Model file for the job. Use its own axes, mm. A direction names the side the tool comes from. Round coordinates to 2 decimals unless told otherwise and drop trailing zeros. Loops run counter-clockwise (first coordinate to the right, second up) from the corner with the lowest first, then second, coordinate; pieces in that order, holes last. Notation, with made-up numbers: M 69.5,34 L 105.5,34 A16 cw 105.5,61 Z; hole C 63.5,-8.5 d6. An arc over 180 degrees is marked long. Use a Markdown table: item, result. Add a question column.
Item 1: Saw through at D-D on z = 6.25. Write the cut outline in (x, y).
Item 2: Saw through at B-B on y = -5. Write the cut outline in (x, z), then the cut area to 3 significant figures.
Item 3: Tool access for faces 4 (the flat face through (8, -46, 5)), 5 (the flat face through (109, -30, 4)): list every direction of +Z, -Z, +X, -X, +Y, -Y with a clear straight run to the whole face (end or side of a thin tool).
Item 4: Saw through at C-C on x = 10.5. Write the cut outline in (y, z).
Item 5: Wall check: L1, parallel to X at y = -36, z = 5.5; L2, parallel to Y at x = 10, z = 4.5; L3, parallel to Y at x = 33, z = 4.5. Give the ranges that are in metal, low to high. Write a range as from..to.
Item 6: Saw through at A-A on z = 1. Write the cut outline in (x, y), then the cut area to 3 significant figures.
Item 7: Pin check, flat tips, straight feed: P1, Ø8, axis at x = 99.5, y = -7.5, coming from the -Z side; P2, Ø3, axis at y = -51, z = 5.5, coming from the -X side; P3, Ø12, axis at x = 39, y = -15, coming from the -Z side. Stop position of each tip, or through.
Item 8: Two-plate mould, pull along Y, no slides. Class faces 1 (the flat face through (54, -59, 4)), 2 (the flat face through (0, -30, 4)), 3 (the flat face through (96, -51, 5)): +Y half, -Y half, draft (parallel to the pull), parting line (faces both ways), or undercut.
```python
from build123d import *

# Parameters (mm, degrees)
ESQUISSE1_W             = 109
ESQUISSE1_H             = 59
BOSS_EXTRU_1_DEPTH      = 9
ESQUISSE2_W             = 103
ESQUISSE2_H             = 53
ENL_V_MAT_EXTRU_1_DEPTH = 8
ESQUISSE3_W             = 10
ESQUISSE3_H             = 10
BOSS_EXTRU_2_DEPTH      = 9
ESQUISSE4_W             = 10
ESQUISSE4_H             = 10
ENL_V_MAT_EXTRU_2_DEPTH = 2


with BuildPart() as part:
    # Esquisse1 → Boss.-Extru.1 (new body)
    with BuildSketch(Plane.XY):
        with Locations((54.5, -29.5)):
            Rectangle(ESQUISSE1_W, ESQUISSE1_H)
    extrude(amount=BOSS_EXTRU_1_DEPTH)

    # Esquisse2 → Enlèv. mat.-Extru.1 (cut)
    with BuildSketch(Plane.XY):
        with Locations((54.5, -29.5)):
            Rectangle(ESQUISSE2_W, ESQUISSE2_H)
    extrude(amount=ENL_V_MAT_EXTRU_1_DEPTH, mode=Mode.SUBTRACT)

    # Esquisse3 → Boss.-Extru.2 (add)
    with BuildSketch(Plane.XY):
        with Locations((101, -8)):
            Rectangle(ESQUISSE3_W, ESQUISSE3_H)
        with Locations((101, -51)):
            Rectangle(ESQUISSE3_W, ESQUISSE3_H)
        with Locations((8, -51)):
            Rectangle(ESQUISSE3_W, ESQUISSE3_H)
        with Locations((8, -8)):
            Rectangle(ESQUISSE3_W, ESQUISSE3_H)
    extrude(amount=BOSS_EXTRU_2_DEPTH)

    # Esquisse4 → Enlèv. mat.-Extru.2 (cut)
    with BuildSketch(Plane.XY):
        with Locations((101, -8)):
            Rectangle(ESQUISSE4_W, ESQUISSE4_H)
        with Locations((101, -51)):
            Rectangle(ESQUISSE4_W, ESQUISSE4_H)
        with Locations((8, -51)):
            Rectangle(ESQUISSE4_W, ESQUISSE4_H)
        with Locations((8, -8)):
            Rectangle(ESQUISSE4_W, ESQUISSE4_H)
    extrude(amount=ENL_V_MAT_EXTRU_2_DEPTH, mode=Mode.SUBTRACT)


solid = part.part
```
Entries:
| question | item | result |
|---|---|---|
| 1 | outline | M 0,-59 L 109,-59 L 109,0 L 0,0 Z; hole M 3,-46 L 13,-46 L 13,-56 L 96,-56 L 96,-46 L 106,-46 L 106,-13 L 96,-13 L 96,-3 L 13,-3 L 13,-13 L 3,-13 Z |
| 2 | outline | M 0,0 L 3,0 L 3,2 L 13,2 L 13,8 L 96,8 L 96,2 L 106,2 L 106,0 L 109,0 L 109,9 L 0,9 Z |
| 2 | area | 277 mm2 |
| 3 | face 4 | -Z |
| 3 | face 5 | +Z, -Z, +X, +Y, -Y |
| 4 | outline | M -59,0 L -56,0 L -56,2 L -46,2 L -46,8 L -13,8 L -13,2 L -3,2 L -3,0 L 0,0 L 0,9 L -59,9 Z |
| 5 | L1 | 0..3, 106..109 |
| 5 | L2 | -59..-46, -13..0 |
| 5 | L3 | -59..-56, -3..0 |
| 6 | outline | M 0,-59 L 109,-59 L 109,0 L 0,0 Z; hole M 3,-56 L 106,-56 L 106,-3 L 3,-3 Z |
| 6 | area | 972 mm2 |
| 7 | P1 | z = 2 |
| 7 | P2 | x = 0 |
| 7 | P3 | z = 8 |
| 8 | face 1 | -Y half |
| 8 | face 2 | draft |
| 8 | face 3 | undercut |
